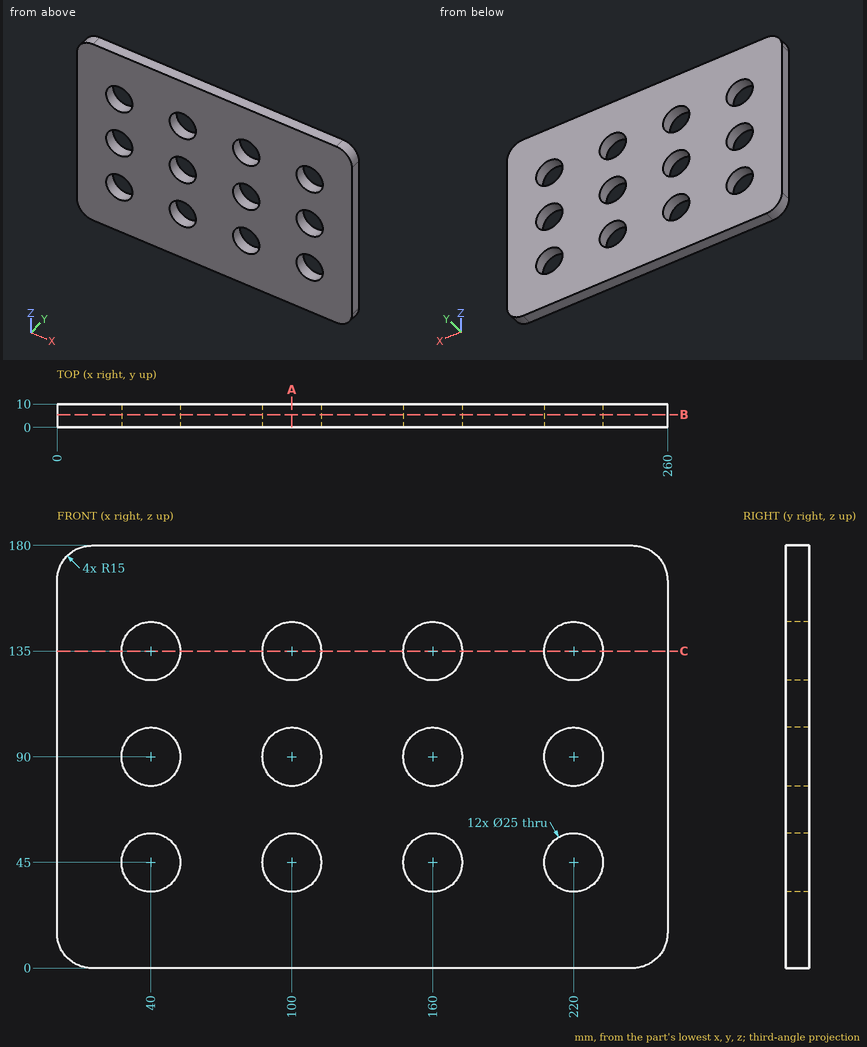
Could you check a few things on this drawing? It's one solid part, dimensions in mm from its lowest x, y, z. Round coordinates to 2 decimals unless told otherwise and drop trailing zeros. Loops run counter-clockwise (first coordinate to the right, second up) from the corner with the lowest first, then second, coordinate; pieces in that order, holes last. Notation, with made-up numbers: M 24.25,41 L 39.25,41 A21 ccw 39.25,45 Z; hole C 43,42.5 d8. An arc over 180 degrees is marked long. Write item = value, one per line. Start each with the question number.
(1) I need wall thicknesses on line 1 along Z through (x, y) = (40, 5); line 2 along X through (y, z) = (4.5, 45); line 3 along Z through (x, y) = (222.5, 8.5). Which ranges of each line are inside material? Lowest first, please.
(2) Suppose I cut it at A-A on x = 100. Write out the boundary of the cut face in (y, z), plus the area to 3 significant figures.
(3) Suppose I cut it at B-B on y = 5.5. Give the number of separate pieces and of enclosed holes in the cut face, plus the area to 3 significant figures.
(4) Suppose I cut it at C-C on z = 135. Write out the boundary of the cut face in (x, y).
Answer block:
q1.line_1 = 0 to 32.5, 57.5 to 77.5, 102.5 to 122.5, 147.5 to 180
q1.line_2 = 0 to 27.5, 52.5 to 87.5, 112.5 to 147.5, 172.5 to 207.5, 232.5 to 260
q1.line_3 = 0 to 32.75, 57.25 to 77.75, 102.25 to 122.75, 147.25 to 180
q2.outline = M 0,0 L 10,0 L 10,32.5 L 0,32.5 Z; M 0,57.5 L 10,57.5 L 10,77.5 L 0,77.5 Z; M 0,102.5 L 10,102.5 L 10,122.5 L 0,122.5 Z; M 0,147.5 L 10,147.5 L 10,180 L 0,180 Z
q2.area = 1,050 mm²
q3.separate_pieces = 1
q3.enclosed_holes = 12
q3.area = 40,700 mm²
q4.outline = M 0,0 L 27.5,0 L 27.5,10 L 0,10 Z; M 52.5,0 L 87.5,0 L 87.5,10 L 52.5,10 Z; M 112.5,0 L 147.5,0 L 147.5,10 L 112.5,10 Z; M 172.5,0 L 207.5,0 L 207.5,10 L 172.5,10 Z; M 232.5,0 L 260,0 L 260,10 L 232.5,10 Z
